Geometry check sheet. Reference: the model listing, model coordinates, mm. Give positions to 0.01 mm unless a question says otherwise; leave off trailing zeros. Order: outer loops, then holes, each group sorted by start corner. A loop starts at its lowest first (then second) coordinate and runs counter-clockwise, first axis right, second up.
from build123d import *

# Parameters (mm, degrees)
SKETCH1_R           = 18.669
BOSS_EXTRUDE1_DEPTH = 57.15
SKETCH2_W           = 6.35
SKETCH2_H           = 1.5875
BOSS_EXTRUDE2_DEPTH = 15.24


with BuildPart() as part:
    # Sketch1 → Boss-Extrude1 (new body)
    with BuildSketch(Plane.XY):
        Circle(SKETCH1_R)
    extrude(amount=BOSS_EXTRUDE1_DEPTH)

    # Sketch2 → Boss-Extrude2 (add)
    with BuildSketch(Plane(origin=(0, 0, 0), x_dir=(-1, 0, 0), z_dir=(0, 0, -1))):
        with Locations((0, 13.9065)):
            Rectangle(SKETCH2_W, SKETCH2_H)
        with Locations((0, -13.9065)):
            Rectangle(SKETCH2_W, SKETCH2_H)
    extrude(amount=BOSS_EXTRUDE2_DEPTH)


solid = part.part
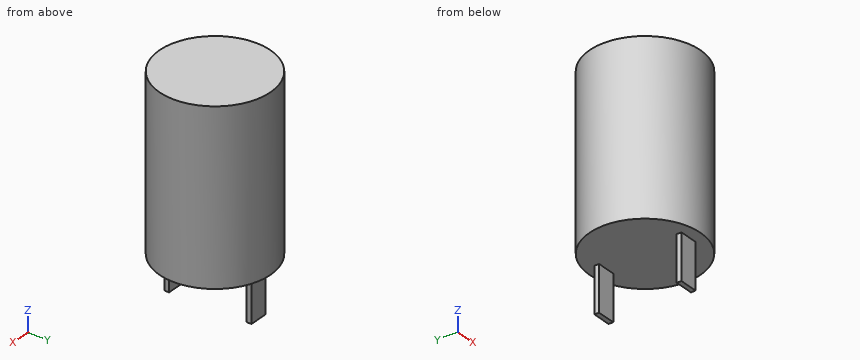
Item 1: Sectioned sample at D-D (z = 4). Enter the section's corners in (x, y).
Reported:
outline: circle Ø37.34 at (0, 0)
Item 2: Sectioned sample at B-B (x = 0). Enter the section's corners in (y, z), and give its area (3 significant figures).
Reported:
outline: (-18.67, 0) - (-14.7, 0) - (-14.7, -15.24) - (-13.11, -15.24) - (-13.11, 0) - (13.11, 0) - (13.11, -15.24) - (14.7, -15.24) - (14.7, 0) - (18.67, 0) - (18.67, 57.15) - (-18.67, 57.15) - close
area: 2,180 mm2
Item 3: Scan lines: L1, parallel to Z at x = 7.5, y = -13; L2, parallel to Y at x = 11, z = 44; L3, parallel to X at y = 16, z = 28.5. Record each from-to range of solid material in increasing order.
Reported:
L1: z = 0 to 57.15
L2: y = -15.08 to 15.08
L3: x = -9.62 to 9.62
Item 4: Gauge pin test, flat ends, axial feed: pin 1 (7 mm diameter, centred on x = 1.5, z = -6.5, fed in from -Y); pin 2 (1.5 mm diameter, centred on y = -11.5, z = 33, fed in from -X); pin 3 (3 mm diameter, centred on x = -0.5, z = -6, fed in from +Y). Record the tip position at first contact, or that the pin passes through.
Reported:
pin 1: stops at y = -14.7
pin 2: stops at x = -15.26
pin 3: stops at y = 14.7
Item 5: Sectioned sample at C-C (y = 0). Enter the section's corners in (x, z).
Reported:
outline: (-18.67, 0) - (18.67, 0) - (18.67, 57.15) - (-18.67, 57.15) - close
Item 6: Sectioned sample at A-A (z = -8.5). Enter the section's corners in (x, y) (3 decimals), and give its area (3 significant figures).
Reported:
outline: (-3.175, -14.7) - (3.175, -14.7) - (3.175, -13.113) - (-3.175, -13.113) - close; (-3.175, 13.113) - (3.175, 13.113) - (3.175, 14.7) - (-3.175, 14.7) - close
area: 20.2 mm2
